Input: part model. Units: mm. Frame: model coordinates. Face numbers are marked on the shaded views. A direction names the side the tool comes from. Round coordinates to 2 decimals unless told otherwise and drop trailing zeros. Order: outer loops, then holes, each group sorted by start corner. A loop starts at its lowest first (then second) coordinate and runs counter-clockwise, first axis right, second up. Notation, with made-up numbers: (84.25, -23.5) -> (93.25, -23.5) arc R12 cw to (93.25, -0.5) -> close; hole circle Ø10 at (63.5, 66). An arc over 180 degrees is marked (long way). Answer as CSV lines item,"result". Start each with the question number.
1) Section query B-B, the plane z = 9.75. Output: boundary loops of the cut face in (x, y).
2) Access query for the marked faces 1, 2 and 3. Directions: +Z, -Z, +X, -X, +Y, -Y. A direction counts if a zero-diameter tool reaches every point of the face in a straight line with its end or side. Return the directions, or none.
3) Line query: L1, parallel to Z at x = 2, y = 3.75; L2, parallel to Z at x = -3.5, y = -2.5; L3, parallel to X at y = -0.5, z = 9. Output: solid intervals per line, ascending.
4) Section query A-A, the plane x = 4.25. Output: boundary loops of the cut face in (y, z), and give its area (3 significant figures).
5) Section query C-C, the plane y = 3.75. Output: boundary loops of the cut face in (x, z).
6) First-contact query: P1, Ø2, axis at y = 0, z = 9, coming from the +X side; P2, Ø6, axis at x = -5, y = 3.5, coming from the -Z side; P3, Ø6, axis at x = -0.5, y = 4, coming from the +Z side; P4, Ø1, axis at x = -4.5, y = -2.5, coming from the +Z side. Flat tips, straight axial feed; report the tip coordinate or a pass-through.
7) Section query D-D, the plane x = -3.75. Output: boundary loops of the cut face in (y, z).
```python
from build123d import *

# Parameters (mm, degrees)
SKETCH_1_R          = 5
EXTRUDE_1_DEPTH     = 4
SKETCH_2_R          = 6
EXTRUDE_2_DEPTH     = 2
SKETCH_3_R          = 5
EXTRUDE_3_DEPTH     = 4
SKETCH_4_R          = 3.5
EXTRUDE_4_DEPTH     = 8
EXTRUDE_START       = 6
SKETCH_5_R          = 3.5
EXTRUDE_5_DEPTH     = 6
CUT_EXTRUDE_START   = -8
CUT_EXTRUDE_2_DEPTH = 8
FILLET_1_R          = 0.5


with BuildPart() as part:
    # 草图1 → 凸台-拉伸1 (new body)
    with BuildSketch(Plane.XY):
        with Locations((-1, 0)):
            Circle(SKETCH_1_R)
    extrude(amount=EXTRUDE_1_DEPTH)

    # 草图2 → 凸台-拉伸2 (add)
    with BuildSketch(Plane(origin=(0, 0, 0), x_dir=(-1, 0, 0), z_dir=(0, 0, -1))):
        Circle(SKETCH_2_R)
    extrude(amount=EXTRUDE_2_DEPTH)

    # 草图3 → 凸台-拉伸3 (add)
    with BuildSketch(Plane(origin=(0, 0, -2), x_dir=(-1, 0, 0), z_dir=(0, 0, -1))):
        with Locations(Location((-1, 0, 0), (0, 0, 179.999112378))):
            Circle(SKETCH_3_R)
    extrude(amount=EXTRUDE_3_DEPTH)

    # 草图4 → 凸台-拉伸4 (add)
    with BuildSketch(Plane.XY.offset(4)):
        Circle(SKETCH_4_R)
    extrude(amount=EXTRUDE_4_DEPTH)

    # 草图5 → 凸台-拉伸5 (add)
    with BuildSketch(Plane(origin=(0, 0, -6), x_dir=(-1, 0, 0), z_dir=(0, 0, -1)).offset(EXTRUDE_START)):
        with Locations(Location((0, 0, 0), (0, 0, 180))):
            Circle(SKETCH_5_R)
    extrude(amount=-EXTRUDE_5_DEPTH)

    # 草图7 → 切除-拉伸2 (cut)
    with BuildSketch(Plane.XY.offset(12).offset(CUT_EXTRUDE_START)):
        with BuildLine():
            ThreePointArc((2.5, -1), (1.767766953, -2.767766953), (0, -3.5))
            ThreePointArc((0, -3.5), (2.474873734, -2.474873734), (3.5, 0))
            ThreePointArc((3.5, 0), (2.47487374, 2.474873729), (1.6e-08, 3.5))
            ThreePointArc((1.6e-08, 3.5), (1.767766959, 2.767766947), (2.5, 1))
            Line((2.5, 1), (2.5, -1))
        make_face()
        with BuildLine():
            ThreePointArc((0, -3.5), (-1.767766953, -2.767766953), (-2.5, -1))
            Line((-2.5, -1), (-2.5, 1))
            ThreePointArc((-2.5, 1), (-1.767766947, 2.767766959), (1.6e-08, 3.5))
            ThreePointArc((1.6e-08, 3.5), (-3.5, 8e-09), (0, -3.5))
        make_face()
    extrude(amount=CUT_EXTRUDE_2_DEPTH, mode=Mode.SUBTRACT)

    # 圆角1
    fillet_1_edges = [part.edges().sort_by_distance(p)[0] for p in [
        (-3.5, 0, -12),
        (0, 3.5, 12),
        (0, -3.5, 12),
        (2.5, 0, 12),
        (-2.5, 0, 12),
    ]]
    fillet(fillet_1_edges, radius=FILLET_1_R)


solid = part.part
```
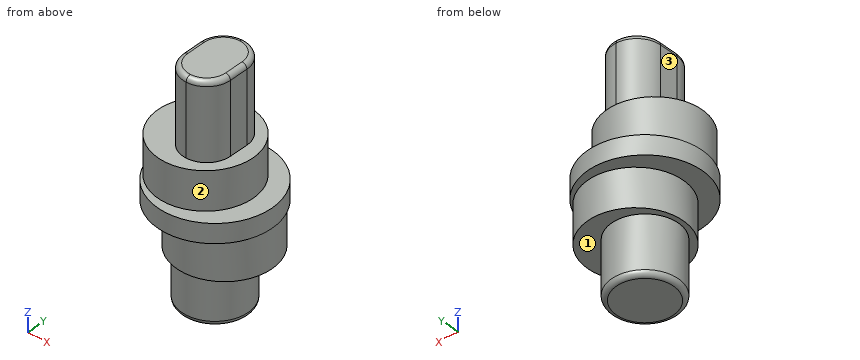
Findings:
1,outline,"(-2.5, -1) arc R2.5 ccw to (2.5, -1) -> (2.5, 1) arc R2.5 ccw to (-2.5, 1) -> close"
2,face 1,"-Z"
2,face 2,"+Z"
2,face 3,"+Z, -X, +Y, -Y"
3,L1,"z = -6 to 4"
3,L2,"z = -2 to 4"
3,L3,"x = -2.5 to 2.5"
4,outline,"(-4.24, -2) -> (-3.8, -2) -> (-3.8, -6) -> (3.8, -6) -> (3.8, -2) -> (4.24, -2) -> (4.24, 0) -> (-4.24, 0) -> close"
4,area,"47.3 mm^2"
5,outline,"(-4.68, -2) -> (-2.31, -2) -> (-2.31, -6) -> (4.31, -6) -> (4.31, -2) -> (4.68, -2) -> (4.68, 0) -> (2.31, 0) -> (2.31, 4) -> (-4.31, 4) -> (-4.31, 0) -> (-4.68, 0) -> close"
6,P1,"stops at x = 2.5"
6,P2,"stops at z = -11.99"
6,P3,"stops at z = 12"
6,P4,"stops at z = 4"
7,outline,"(-4.68, -2) -> (-1.56, -2) -> (-1.56, -6) -> (1.56, -6) -> (1.56, -2) -> (4.68, -2) -> (4.68, 0) -> (4.18, 0) -> (4.18, 4) -> (-4.18, 4) -> (-4.18, 0) -> (-4.68, 0) -> close"
